Design review of the part built by this model. Coordinates are the model's own, in mm. Face numbers are marked on the shaded views. A direction names the side the tool comes from. Coordinates: 2 decimals unless noted, no trailing zeros. Write each loop counter-clockwise with the first axis right and the second up, starting at its lowest first coordinate (ties: lowest second). Pieces come first, ordered by that corner, then holes. Notation, with made-up numbers: M 63,27.25 L 84,27.25 A20 cw 84,51.25 Z; hole C 68,-21 d2. An arc over 180 degrees is marked long. Write item = value, one per line.
```python
from build123d import *

# Parameters (mm, degrees)
F0_W          = 16
F0_H          = 25
F1_DEPTH      = 9
F2_T          = -2
F4_DEPTH      = 6
F5_R          = 1.625
F6_DEPTH      = 25
F7_R          = 1.125
F8_DEPTH      = 25
F8_DEPTH_BACK = 25
F9_R          = 1
F11_W         = 3.5
F11_H         = 6
F11_W_2       = 2
F11_H_2       = 4
F12_DEPTH     = 2.5
F13_R         = 1
F14_R         = 0.25
F15_SIZE2     = 1.3737387097
F15_SIZE      = 0.5
F16_R         = 0.5
F17_R         = 0.5


# Not quite as in the source:
# - two fillets or chamfers of one size are made in one step


with BuildPart() as f1:
    # F0 (on Top) → F1 (new body)
    with BuildSketch(Plane.XY):
        Rectangle(F0_W, F0_H)
    extrude(amount=-F1_DEPTH)

    # F2
    f2_openings = [f1.faces().sort_by_distance(p)[0] for p in [
        (0, 0, 0),
    ]]
    offset(amount=F2_T, openings=f2_openings)

    # F3 (on Front) → F4 (join, symmetric)
    with BuildSketch(Plane.XZ):
        with BuildLine():
            ThreePointArc((-9, 1.5), (-12.0919927986, 3.7641877852), (-13.3170916435, 0.1329209796))
            Line((-13.3170916435, 0.1329209796), (-9, -6))
            Line((-9, -6), (-8, -6))
            Line((-8, -6), (-8, 0))
            Line((-8, 0), (-9, 0))
            Line((-9, 0), (-9, 1.5))
        make_face()
    extrude(amount=F4_DEPTH, both=True)

    # F5 (on face) → F6 (cut)
    with BuildSketch(Plane(origin=(0, 6, 0), x_dir=(-1, 0, 0), z_dir=(0, 1, 0))):
        with Locations((11.375, 1.5)):
            Circle(F5_R)
    extrude(amount=-F6_DEPTH, mode=Mode.SUBTRACT)

    # F7 (on Front) → F8 (cut, two sides)
    with BuildSketch(Plane.XZ) as f8_sk:
        Circle(F7_R)
    extrude(amount=-F8_DEPTH, mode=Mode.SUBTRACT)
    extrude(f8_sk.sketch, amount=F8_DEPTH_BACK, mode=Mode.SUBTRACT)

    # F9
    f9_edges = [f1.edges().sort_by_distance(p)[0] for p in [
        (8, -12.5, -4.5),
        (8, 12.5, -4.5),
        (-8, -12.5, -4.5),
        (-8, 12.5, -4.5),
        (-9, 0, -6),
    ]]
    fillet(f9_edges, radius=F9_R)

    # F11 (on face) → F12 (join)
    with BuildSketch(Plane.XY):
        with Locations((9.75, 0)):
            Rectangle(F11_W, F11_H)
        with Locations((9.25, 0)):
            Rectangle(F11_W_2, F11_H_2, mode=Mode.SUBTRACT)
    extrude(amount=-F12_DEPTH)

    # F13
    f13_edges = [f1.edges().sort_by_distance(p)[0] for p in [
        (11.5, -3, -1.25),
        (8, -3, -1.25),
        (11.5, 3, -1.25),
        (8, 3, -1.25),
    ]]
    fillet(f13_edges, radius=F13_R)

    # F14
    f14_edges = [f1.edges().sort_by_distance(p)[0] for p in [
        (9.25, 2, 0),
        (8.25, 0, 0),
        (9.25, -2, 0),
    ]]
    fillet(f14_edges, radius=F14_R)

    # F15
    f15_edges = [f1.edges().sort_by_distance(p)[0] for p in [
        (10.25, 0, 0),
    ]]
    f15_side = f1.faces().sort_by_distance((6.594217, 0, 0))[0]
    chamfer(f15_edges, length=F15_SIZE, length2=F15_SIZE2, reference=f15_side)

    # F16
    f16_edges = [f1.edges().sort_by_distance(p)[0] for p in [
        (0, 12.5, -1.125),
        (0, -12.5, -1.125),
    ]]
    fillet(f16_edges, radius=F16_R)

    # F17
    f17_edges = [f1.edges().sort_by_distance(p)[0] for p in [
        (0, 10.5, -1.125),
        (0, 10.5, -7),
        (0, -10.5, -7),
        (6, 0, -7),
        (0, -10.5, -1.125),
        (-6, 0, -7),
    ]]
    fillet(f17_edges, radius=F17_R)


solid = f1.part
```
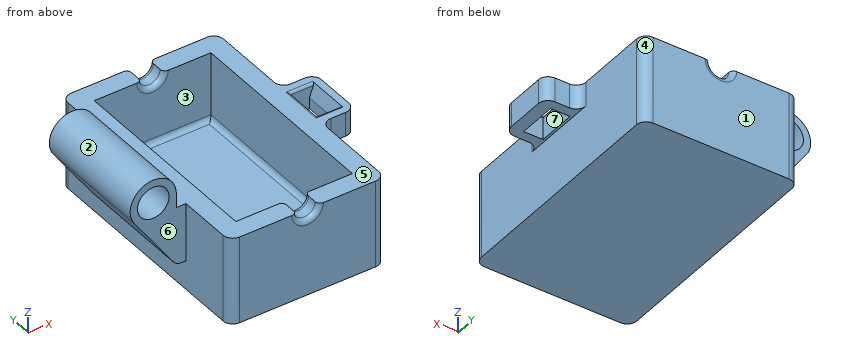
Q1. The part is to be moulded in two halves that separate along X. For the marked faces 1, 2, 3 and 4, say which applies: +X half, -X half, draft (parallel to the pull), parting line (faces both ways), or undercut.
Check result:
face_1 = draft
face_2 = parting line
face_3 = undercut
face_4 = +X half
Q2. Consider section C-C, the plane z = 1. State the section outline as (x, y) points.
Check result:
outline = M -13.7,-6 L -12.92,-6 L -12.92,6 L -13.7,6 Z; M -9.83,-6 L -9,-6 L -9,6 L -9.83,6 Z
Q3. Consider section D-D, the plane x = -11.5. State the section outline as (y, z) points, and give its area (3 significant figures).
Check result:
outline = M -6,-2.45 L 6,-2.45 L 6,-0.12 L -6,-0.12 Z; M -6,3.12 L 6,3.12 L 6,3.87 L -6,3.87 Z
area = 37.0 mm²
Q4. Wall thickness on line 1 (Y direction, x = 9.25, z = -1.5); line 2 (X direction, y = -6.5, z = -4.75); line 3 (Y direction, x = -9.5, z = -1.5): over which ranges is each line inside the solid? List them lowest first.
Check result:
line_1 = -3 to -2, 2 to 3
line_2 = -8 to -6, 6 to 8
line_3 = -6 to 6
Q5. For P1, Ø1, axis at x = 10, y = -1, coming from the -Z side; P2, Ø9, axis at x = 2, y = 3.5, coming from the +Z side; P3, Ø1, axis at x = -9.5, y = -5.5, coming from the -Z side, all flat-tipped, find the tip position at first contact; note any pin that passes through.
Check result:
P1 = -2.5
P2 = 0
P3 = -5.85
Q6. Machinability: for the marked faces 5, 6 and 7, which of the approach directions +Z, -Z, +X, -X, +Y, -Y give a long, thin tool a straight path to every point of the face, cutting with its end or side? Answer none if there is none.
Check result:
face_5 = +Z, +X, +Y, -Y
face_6 = +Z, -Z, -X, -Y
face_7 = +Z, -Z
Q7. Consider section A-A, the plane y = -1. State the section outline as (x, z) points (3 decimals).
Check result:
outline = M -13.317,0.133 L -9.299,-5.576 A1 ccw -8.481,-6 L -8,-6 L -8,-9 L 8,-9 L 8,-2.5 L 8.25,-2.5 L 8.25,-0.25 A0.25 ccw 8,0 L 6,0 L 6,-6.5 A0.5 cw 5.5,-7 L -5.5,-7 A0.5 cw -6,-6.5 L -6,0 L -9,0 L -9,1.5 A2.375 ccw long Z; M 10.25,-2.5 L 11.5,-2.5 L 11.5,0 L 10.75,0 L 10.25,-1.374 Z; hole C -11.375,1.5 d3.25
Q8. Consider section B-B, the plane x = 0. State the section outline as (y, z) points (3 decimals).
Check result:
outline = M -12.5,-9 L 12.5,-9 L 12.5,-1.625 A0.5 ccw 12,-1.125 L 11,-1.125 A0.5 ccw 10.5,-1.625 L 10.5,-6.5 A0.5 cw 10,-7 L -10,-7 A0.5 cw -10.5,-6.5 L -10.5,-1.625 A0.5 ccw -11,-1.125 L -12,-1.125 A0.5 ccw -12.5,-1.625 Z
